from build123d import *

# Parameters (mm, degrees)
BOSS_EXTRUDE1_DEPTH = 511
CUT_EXTRUDE1_DEPTH  = 23


with BuildPart() as part:
    # Sketch1 → Boss-Extrude1 (new body)
    with BuildSketch(Plane.XY):
        Polygon((0, 0), (20, 0), (20, 2), (2, 2), (2, 20), (0, 20), align=None)
    extrude(amount=BOSS_EXTRUDE1_DEPTH)

    # Sketch2 → Cut-Extrude1 (cut, symmetric)
    with BuildSketch(Plane(origin=(0, 2, 0), x_dir=(1, 0, 0), z_dir=(0, 1, 0))):
        Polygon((0, -511), (20, -511), (0, -491), align=None)
        Polygon((20, 0), (0, -20), (0, 0), align=None)
    extrude(amount=CUT_EXTRUDE1_DEPTH, both=True, mode=Mode.SUBTRACT)


solid = part.part
Here's how the part is built. I have some questions about the finished solid (model axes, mm). A direction names the side the tool comes from. Round coordinates to 2 decimals unless told otherwise and drop trailing zeros. Write each loop counter-clockwise with the first axis right and the second up, starting at its lowest first coordinate (ties: lowest second). Pieces come first, ordered by that corner, then holes.
1. Will this pin go through, and if not, where does the flat tip stop? pin 1 Ø2 at (x, z) = (16.5, 250.5) entering from +Y.
2. For faces 1 (the flat face through (0, 10, 252)), 2 (the flat face through (2, 11, 252)), which set-ups out of +Z, -Z, +X, -X, +Y, -Y let a thin tool reach every point of the face, with its end or its side?
3. I need wall thicknesses on L1, parallel to Y at x = 18, z = 278.5; L2, parallel to Z at x = 17, y = 1. Which ranges of each line are inside material? Lowest first, please.
4. Suppose I cut it at C-C (y = 5.75). List the corners of the cut face in (x, z) for me.
5. Suppose I cut it at A-A (z = 257). List the corners of the cut face in (x, y) for me, and give its area (3 significant figures).
6. Suppose I cut it at B-B (x = 9.75). List the corners of the cut face in (y, z) for me.
Answer sheet:
1. pin 1: stops at y = 2
2. face 1: +Z, -Z, -X, +Y, -Y
2. face 2: +Z, -Z, +X, +Y
3. L1: y = 0 to 2
3. L2: z = 3 to 508
4. outline: (0, 20) - (2, 18) - (2, 493) - (0, 491) - close
5. outline: (0, 0) - (20, 0) - (20, 2) - (2, 2) - (2, 20) - (0, 20) - close
5. area: 76.0 mm2
6. outline: (0, 10.25) - (2, 10.25) - (2, 500.75) - (0, 500.75) - close
